```python
from build123d import *

# Parameters (mm, degrees)
BODY_DEPTH                         = 6.35
HANDLE_DEPTH                       = 6.35
SKETCH3_R                          = 10
BEARING_RINGS_DEPTH                = 3.175
SKETCH7_W                          = 239.992041534
SKETCH7_H                          = 70
OUTSIDE_PERIMETER_CONSTRAINT_DEPTH = 7.5
SKETCH10_W                         = 200
SKETCH10_H                         = 50
INSIDE_PERIMETER_CONSTRAINT_DEPTH  = 7.5
SKETCH11_R                         = 5
LOCKING_MECHANISM_HOLES_DEPTH      = 6.36
SKETCH12_W                         = 45
SKETCH12_H                         = 45
SQUARE_BEARING_CUT_DEPTH           = 6.35
FILLET1_R                          = 40
FILLET2_R                          = 40


with BuildPart() as part:
    # Sketch1 → Body (new body)
    with BuildSketch(Plane(origin=(0, 0, 0), x_dir=(1, 0, 0), z_dir=(0, 1, 0))):
        Polygon((0, 0), (294, 0), (336.996020767, 43.003978862), (336.996020767, 337.003978862), (217, 456.999999629), (77, 456.999999629), (-42.996020767, 337.003978862), (-42.996020767, 43.003978862), align=None)
    extrude(amount=BODY_DEPTH)

    # Sketch2 → Handle (cut)
    with BuildSketch(Plane(origin=(0, 6.35, 0), x_dir=(1, 0, 0), z_dir=(0, 1, 0))):
        with BuildLine():
            Line((112.35, 441.799999629), (181.65, 441.799999629))
            ThreePointArc((181.65, 441.799999629), (197.5, 425.949999629), (181.65, 410.099999629))
            Line((181.65, 410.099999629), (112.35, 410.099999629))
            ThreePointArc((112.35, 410.099999629), (96.5, 425.949999629), (112.35, 441.799999629))
        make_face()
    extrude(amount=-HANDLE_DEPTH, mode=Mode.SUBTRACT)

    # Sketch3 → Bearing Rings (cut)
    with BuildSketch(Plane(origin=(0, 6.35, 0), x_dir=(1, 0, 0), z_dir=(0, 1, 0))):
        with Locations(Location((27.003979233, 300, 0), (0, 0, 270))):
            Circle(SKETCH3_R)
        with Locations(Location((266.996020767, 300, 0), (0, 0, 270))):
            Circle(SKETCH3_R)
        with Locations(Location((266.996020767, 50, 0), (0, 0, 270))):
            Circle(SKETCH3_R)
        with Locations(Location((27.003979233, 50, 0), (0, 0, 270))):
            Circle(SKETCH3_R)
    extrude(amount=-BEARING_RINGS_DEPTH, mode=Mode.SUBTRACT)

    # Sketch7 → Outside Perimeter Constraint (add)
    with BuildSketch(Plane(origin=(0, 6.35, 0), x_dir=(1, 0, 0), z_dir=(0, 1, 0))):
        with Locations((147, 175)):
            Rectangle(SKETCH7_W, SKETCH7_H)
    extrude(amount=OUTSIDE_PERIMETER_CONSTRAINT_DEPTH)

    # Sketch10 → Inside Perimeter Constraint (cut)
    with BuildSketch(Plane(origin=(0, 13.85, 0), x_dir=(1, 0, 0), z_dir=(0, 1, 0))):
        with Locations((147, 175)):
            Rectangle(SKETCH10_W, SKETCH10_H)
    extrude(amount=-INSIDE_PERIMETER_CONSTRAINT_DEPTH, mode=Mode.SUBTRACT)

    # Sketch11 → Locking Mechanism Holes (cut)
    with BuildSketch(Plane(origin=(0, 6.35, 0), x_dir=(1, 0, 0), z_dir=(0, 1, 0))):
        with Locations(Location((221.65, 421.999999629, 0), (0, 0, 270))):
            Circle(SKETCH11_R)
        with Locations(Location((72.35, 421.999999629, 0), (0, 0, 270))):
            Circle(SKETCH11_R)
    extrude(amount=-LOCKING_MECHANISM_HOLES_DEPTH, mode=Mode.SUBTRACT)

    # Sketch12 → Square Bearing Cut (cut)
    with BuildSketch(Plane(origin=(0, 6.35, 0), x_dir=(1, 0, 0), z_dir=(0, 1, 0))):
        with Locations((34.503979233, 289.499999629)):
            Rectangle(SKETCH12_W, SKETCH12_H)
        with Locations((259.496020767, 289.499999629)):
            Rectangle(SKETCH12_W, SKETCH12_H)
        with Locations((259.496020767, 60.500000371)):
            Rectangle(SKETCH12_W, SKETCH12_H)
        with Locations((34.503979233, 60.500000371)):
            Rectangle(SKETCH12_W, SKETCH12_H)
    extrude(amount=-SQUARE_BEARING_CUT_DEPTH, mode=Mode.SUBTRACT)

    # Fillet1
    fillet1_edges = [part.edges().sort_by_distance(p)[0] for p in [
        (77, 3.175, -456.999999629),
        (217, 3.175, -456.999999629),
    ]]
    fillet(fillet1_edges, radius=FILLET1_R)

    # Fillet2
    fillet2_edges = [part.edges().sort_by_distance(p)[0] for p in [
        (-42.996020767, 3.175, -43.003978862),
        (-42.996020767, 3.175, -337.003978862),
        (336.996020767, 3.175, -337.003978862),
        (336.996020767, 3.175, -43.003978862),
        (294, 3.175, 0),
        (0, 3.175, 0),
    ]]
    fillet(fillet2_edges, radius=FILLET2_R)


solid = part.part
```
Geometry check sheet. Reference: the model listing, model coordinates, mm. A direction names the side the tool comes from. Round coordinates to 2 decimals unless told otherwise and drop trailing zeros. Order: outer loops, then holes, each group sorted by start corner. A loop starts at its lowest first (then second) coordinate and runs counter-clockwise, first axis right, second up. Notation, with made-up numbers: (19, 51) - (64, 51) arc R18 cw to (64, 85) - close; hole circle Ø5 at (-1, 2). An arc over 180 degrees is marked (long way). Use a Markdown table: item, result. Add a question column.
1) Section check C-C (x = 125.5). Record the cut outline in (y, z).
2) Gauge pin test, flat ends, axial feed: P1, Ø4, axis at y = 9.5, z = -170.5, coming from the +X side; P2, Ø4, axis at x = 7.5, z = -183, coming from the +Y side; P3, Ø3, axis at x = 263.5, y = 3.5, coming from the -Z side; P4, Ø12, axis at x = 67.5, z = -77, coming from the -Y side. Record the tip position at first contact, or that the pin passes through.
3) Section check D-D (z = -191). Record the cut outline in (x, y).
4) Set-up check for faces 5 (the flat face through (146, 6.35, -175)), 6 (the cylindrical face through (215.94, 3.22, -453.87)): record each of +Z, -Z, +X, -X, +Y, -Y from which the full face is reachable in a straight line by a thin tool's end or side.
5) Mould release check, pull along X, two halves, no side actions. Record for faces 1 (the flat face through (145, 13.85, -144)), 2 (the cylindrical face through (96.504, 3.219, -425.601)), 3 (the cylindrical face through (197.496, 3.219, -426.299)), 4 (the cylindrical face through (-39.866, 3.219, -335.946)): released by +X, released by -X, zero draft, split by the parting line, or undercut.
6) Section check A-A (y = 9). Record the cut outline in (x, z), then the cut area to 3 significant figures.
7) Thickness scan on line 1 along X through (y, z) = (5.5, -295); line 2 along X through (y, z) = (10.25, -183); line 3 along Z through (x, y) = (70, 10.5). Record the ranges inside material, lowest first.
8) Section check B-B (z = -306.5). Record the cut outline in (x, y).
Established:
| question | item | result |
|---|---|---|
| 1 | outline | (0, -457) - (6.35, -457) - (6.35, -441.8) - (0, -441.8) - close; (0, -410.1) - (6.35, -410.1) - (6.35, -210) - (13.85, -210) - (13.85, -200) - (6.35, -200) - (6.35, -150) - (13.85, -150) - (13.85, -140) - (6.35, -140) - (6.35, 0) - (0, 0) - close |
| 2 | P1 | x = 267 |
| 2 | P2 | y = 6.35 |
| 2 | P3 | z = -412 |
| 2 | P4 | y = 0 |
| 3 | outline | (-43, 0) - (337, 0) - (337, 6.35) - (267, 6.35) - (267, 13.85) - (247, 13.85) - (247, 6.35) - (47, 6.35) - (47, 13.85) - (27, 13.85) - (27, 6.35) - (-43, 6.35) - close |
| 4 | face 5 | +Y |
| 4 | face 6 | -Z, +X, +Y, -Y |
| 5 | face 1 | zero draft |
| 5 | face 2 | undercut |
| 5 | face 3 | undercut |
| 5 | face 4 | released by -X |
| 6 | outline | (27, -210) - (267, -210) - (267, -140) - (27, -140) - close; hole (47, -200) - (247, -200) - (247, -150) - (47, -150) - close |
| 6 | area | 6,800 mm2 |
| 7 | line 1 | -43 to 12, 57 to 237, 282 to 337 |
| 7 | line 2 | 27 to 47, 247 to 267 |
| 7 | line 3 | -210 to -200, -150 to -140 |
| 8 | outline | (-43, 0) - (12, 0) - (12, 6.35) - (-43, 6.35) - close; (57, 0) - (237, 0) - (237, 6.35) - (57, 6.35) - close; (282, 0) - (337, 0) - (337, 6.35) - (282, 6.35) - close |
